from build123d import *

# Parameters (mm, degrees)
F0_R     = 8.053641
F1_DEPTH = 50.8
F2_SIZE  = 1.27
F3_SIZE  = 1.27
F4_W     = 2.679992
F4_H     = 2.559151
F5_DEPTH = 9.144


with BuildPart() as f1:
    # F0 (on Top) → F1 (new body)
    with BuildSketch(Plane.XY):
        Circle(F0_R)
    extrude(amount=F1_DEPTH)

    # F2
    f2_edges = [f1.edges().sort_by_distance(p)[0] for p in [
        (-8.053641, 0, 50.8),
    ]]
    chamfer(f2_edges, length=F2_SIZE)

    # F3
    f3_edges = [f1.edges().sort_by_distance(p)[0] for p in [
        (-8.053641, 0, 0),
    ]]
    chamfer(f3_edges, length=F3_SIZE)

    # F4 (on Front) → F5 (join)
    with BuildSketch(Plane.XZ):
        with Locations((0, 22.032296)):
            Rectangle(F4_W, F4_H)
    extrude(amount=F5_DEPTH)


solid = f1.part
Geometry: final body of the model. Coordinates: model frame, mm. A direction names the side the tool comes from. Coordinates: 2 decimals unless noted, no trailing zeros. Order: outer loops, then holes, each group sorted by start corner. A loop starts at its lowest first (then second) coordinate and runs counter-clockwise, first axis right, second up. Notation, with made-up numbers: M 57.25,-17.5 L 97.25,-17.5 A38 cw 97.25,20.5 Z; hole C 84.5,-31.5 d2. An arc over 180 degrees is marked long. One line per question, with ' | ' between items. Start each with the question number.
Item 1: Cut plane B-B, the plane z = 36. Return the cut outline in (x, y), then the cut area to 3 significant figures.
Item 2: Ray query, probe 1 along Y at (x, z) = (0.5, 8); probe 2 along X at (y, z) = (-3, 34); probe 3 along X at (y, z) = (-3.5, 38.5). Return the intervals inside material, ascending. Write a range as [from, to].
Item 3: Cut plane A-A, the plane x = 0. Return the cut outline in (y, z).
Item 4: Set-up query: faces 1 (the flat face through (1.34, -8.5, 22)), 2 (the flat face through (0, 0, 50.8)), 3 (the flat face through (-1.34, -8.5, 22)). Return all of +Z, -Z, +X, -X, +Y, -Y with unobstructed straight access to the full face (end or side cutting, diameter ignored); none if empty.
Item 5: Pin query (flat end, axial travel): pin 1 Ø0.6 at (x, y) = (0, -8.5) entering from -Z; pin 2 Ø5 at (x, z) = (1, 32) entering from -Y; pin 3 Ø3 at (x, z) = (-3, 21.5) entering from +Y. Return the tip coordinate at first contact, or that it passes through.
A:
1) outline: C 0,0 d16.11 | area: 204 mm2
2) probe 1: y = [-8.04, 8.04] | probe 2: x = [-7.47, 7.47] | probe 3: x = [-7.25, 7.25]
3) outline: M -9.14,20.75 L -8.05,20.75 L -8.05,1.27 L -6.78,0 L 6.78,0 L 8.05,1.27 L 8.05,49.53 L 6.78,50.8 L -6.78,50.8 L -8.05,49.53 L -8.05,23.31 L -9.14,23.31 Z
4) face 1: +Z, -Z, +X, -Y | face 2: +Z, +X, -X, +Y, -Y | face 3: +Z, -Z, -X, -Y
5) pin 1: stops at z = 20.75 | pin 2: stops at y = -8.05 | pin 3: stops at y = 7.91
